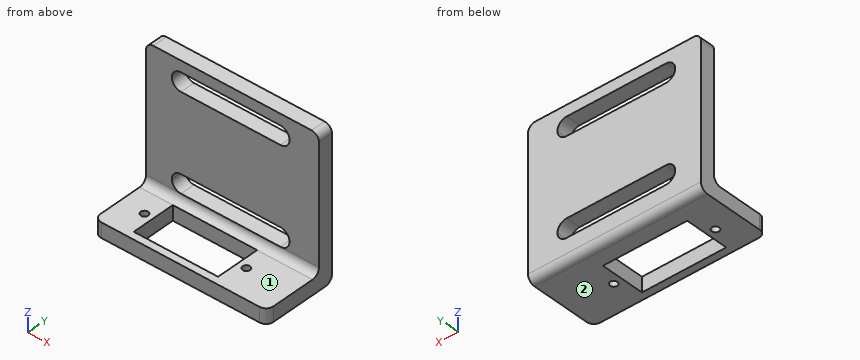
Autodesk Fusion 360 part; units mm, degrees
sketch "Sketch1" plane through (0, 0, 0) normal (0, 0, 1) x (1, 0, 0)
  line L0 (31.95, 2) -> (31.95, 14)
  line L1 (0, 20) -> (0, 0)
  line L2 (47, 0) -> (47, 20)
  line L3 (4.25, 2) -> (4.25, 14)
  line L4 (47, 16) -> (0, 16)
  line L5 (4.25, 14) -> (36.75, 14)
  line L6 (0, 16) -> (0, 20)
  line L7 (36.75, 14) -> (36.75, 2)
  line L8 (47, 20) -> (47, 16)
  line L9 (4.25, 14) -> (4.25, 2)
  line L10 (36.75, 2) -> (4.25, 2)
  line L11 (47, 20) -> (0, 20)
  line L12 (0, 0) -> (47, 0)
  circle A0 centre (34.35, 8) radius 1
  circle A1 centre (6.65, 8) radius 1
  line L13 (4.25, 2) -> (9.05, 2)
  line L14 (36.75, 14) -> (36.75, 2)
  line L15 (31.95, 14) -> (36.75, 14)
  line L16 (9.05, 14) -> (4.25, 14)
  line L17 (9.05, 2) -> (9.05, 14)
  line L18 (0, 20) -> (47, 20)
  line L19 (36.75, 2) -> (31.95, 2)
  dimension "d1" = 47
  dimension "d2" = 20
  dimension "d5" = 4
  dimension "d20" = 32.5
  dimension "d21" = 12
  dimension "d22" = 4.8
  dimension "d23" = 4.8
  dimension "d24" = 2
  dimension "d25" = 2
extrude "Extrude1" add sketch "Sketch1" along normal blind 4 contours L0 L5 L7 L10 L14 L15 L19 | L3 L5 L9 L10 L13 L16 L17 | L1 L2 L4 L12
extrude "Extrude2" add sketch "Sketch1" along normal blind 28 contours L1 L2 L4 L6 L8 L11 L18
extrude "Extrude3" add 1 faces at (15.6667, 18.6667, 28) along direction (0, 0, 1) blind 12
ref_plane "WorkPlane1" through (23.5, 18, 37) normal (0, 0, 1) x (1, 0, 0)
sketch "Sketch2" plane through (20, 18, 37) normal (0, 0, 1) x (1, 0, 0)
  line L0 (-13, -3) -> (19, -3)
  line L1 (19, -3) -> (19, 5)
  line L2 (19, 5) -> (-13, 5)
  line L3 (-13, 5) -> (-13, -3)
extrude "Extrude4" cut sketch "Sketch2" against normal blind 5
ref_plane "WorkPlane2" through (23, 18, 11) normal (0, 0, 1) x (1, 0, 0)
sketch "Sketch3" plane through (20, 18, 11) normal (0, 0, 1) x (1, 0, 0)
  line L0 (-13, -3) -> (19, -3)
  line L1 (19, -3) -> (19, 5)
  line L2 (19, 5) -> (-13, 5)
  line L3 (-13, 5) -> (-13, -3)
extrude "Extrude5" cut sketch "Sketch3" against normal blind 5
fillet "Fillet1" radius 2.5 8 edges at (7, 18, 6) (7, 18, 11) (39, 18, 11) (39, 18, 6) (39, 18, 32) (39, 18, 37) (7, 18, 37) (7, 18, 32)
fillet "Fillet2" radius 2 6 edges at (47, 18, 40) (0, 18, 40) (23.5, 16, 4) (47, 0, 2) (0, 0, 2) (23.5, 20, 0)
Check sheet for the modelled part. Datum: model origin and axes. Units: mm. Face numbers are marked on the shaded views. A direction names the side the tool comes from. Give positions to 0.01 mm unless a question says otherwise; leave off trailing zeros. Write each loop counter-clockwise with the first axis right and the second up, starting at its lowest first coordinate (ties: lowest second). Pieces come first, ordered by that corner, then holes.
Item 1: Cross-section at B-B (y = 11). Enter the section's corners in (x, z).
Item 2: Access from +Z, -Z, +X, -X, +Y, -Y to the whole of each face (thin tool, end or side, straight path). Record for the marked faces 1 and 2.
Item 3: Scan lines: L1, parallel to Z at x = 18.5, y = 17; L2, parallel to Z at x = 16.5, y = 19.25; L3, parallel to Y at x = 34.35, z = 2.5. Record each from-to range of solid material in increasing order.
Item 4: Gauge pin test, flat ends, axial feed: pin 1 (2.5 mm diameter, centred on x = 6.65, y = 8, fed in from +Z); pin 2 (10 mm diameter, centred on x = 14, z = 8.5, fed in from -Y); pin 3 (4 mm diameter, centred on x = 33, z = 17, fed in from -Y). Record the tip position at first contact, or that the pin passes through.
Item 5: Cross-section at D-D (z = 7.5). Enter the section's corners in (x, y), and give its area (3 significant figures).
Item 6: Cross-section at A-A (x = 28). Count the separate pieces of the cut face and the enclosed holes in it, and give its area (3 significant figures).
Item 7: Cross-section at C-C (y = 8). Enter the section's corners in (x, z), and give its area (3 significant figures).
Report:
1. outline: (0, 0) - (9.05, 0) - (9.05, 4) - (0, 4) - close; (31.95, 0) - (47, 0) - (47, 4) - (31.95, 4) - close
2. face 1: +Z, +X, -X, -Y
2. face 2: -Z, +X, -X, +Y, -Y
3. L1: z = 0 to 6, 11 to 32, 37 to 40
3. L2: z = 0.44 to 6, 11 to 32, 37 to 40
3. L3: y = 0 to 7, 9 to 20
4. pin 1: stops at z = 4
4. pin 2: stops at y = 0
4. pin 3: stops at y = 16
5. outline: (0, 16) - (7.21, 16) - (7.21, 20) - (0, 20) - close; (38.79, 16) - (47, 16) - (47, 20) - (38.79, 20) - close
5. area: 61.7 mm2
6. separate pieces: 4
6. enclosed holes: 0
6. area: 136 mm2
7. outline: (0, 0) - (5.65, 0) - (5.65, 4) - (0, 4) - close; (7.65, 0) - (9.05, 0) - (9.05, 4) - (7.65, 4) - close; (31.95, 0) - (33.35, 0) - (33.35, 4) - (31.95, 4) - close; (35.35, 0) - (47, 0) - (47, 4) - (35.35, 4) - close
7. area: 80.4 mm2
